Input: dimensioned drawing with shaded views. Units: mm. Origin: part minimum x, y, z. Coordinates: 2 decimals unless noted, no trailing zeros. Loops run counter-clockwise (first coordinate to the right, second up) from the corner with the lowest first, then second, coordinate; pieces in that order, holes last. Notation, with made-up numbers: (29, 4.5) - (67, 4.5) arc R22 cw to (67, 11.5) - close; hole circle Ø9 at (-2, -5). An arc over 180 degrees is marked (long way). Put each result on its own line as item: value. Start each with the question number.
1) Material intervals for line 1 along Y through (x, z) = (15.5, 6); line 2 along X through (y, z) = (7.5, 8.75); line 3 along Z through (x, y) = (13.5, 38), sorted ascending. Write a range as from..to.
2) Section B-B on z = 7.25. Output: boundary loops of the cut face in (x, y), and give its area (4 significant figures).
3) Section C-C on x = 2. Output: boundary loops of the cut face in (y, z).
4) Draft query along Z for the marked faces 1, 2 and 3. Return one class per face: +Z half, -Z half, draft (parallel to the pull), parting line (faces both ways), or undercut.
5) Section A-A on x = 9.25. Output: boundary loops of the cut face in (y, z).
6) Section D-D on z = 11. Output: boundary loops of the cut face in (x, y), and give its area (3 significant figures).
7) Contact query for flat-ended pins moving along their axis: pin 1 Ø5 at (x, z) = (18, 11.5) entering from -Y; pin 2 Ø1.5 at (x, z) = (8, 9) entering from +Y; pin 3 Ø4 at (y, z) = (6, 4) entering from -X. Output: stop coordinate, or through.
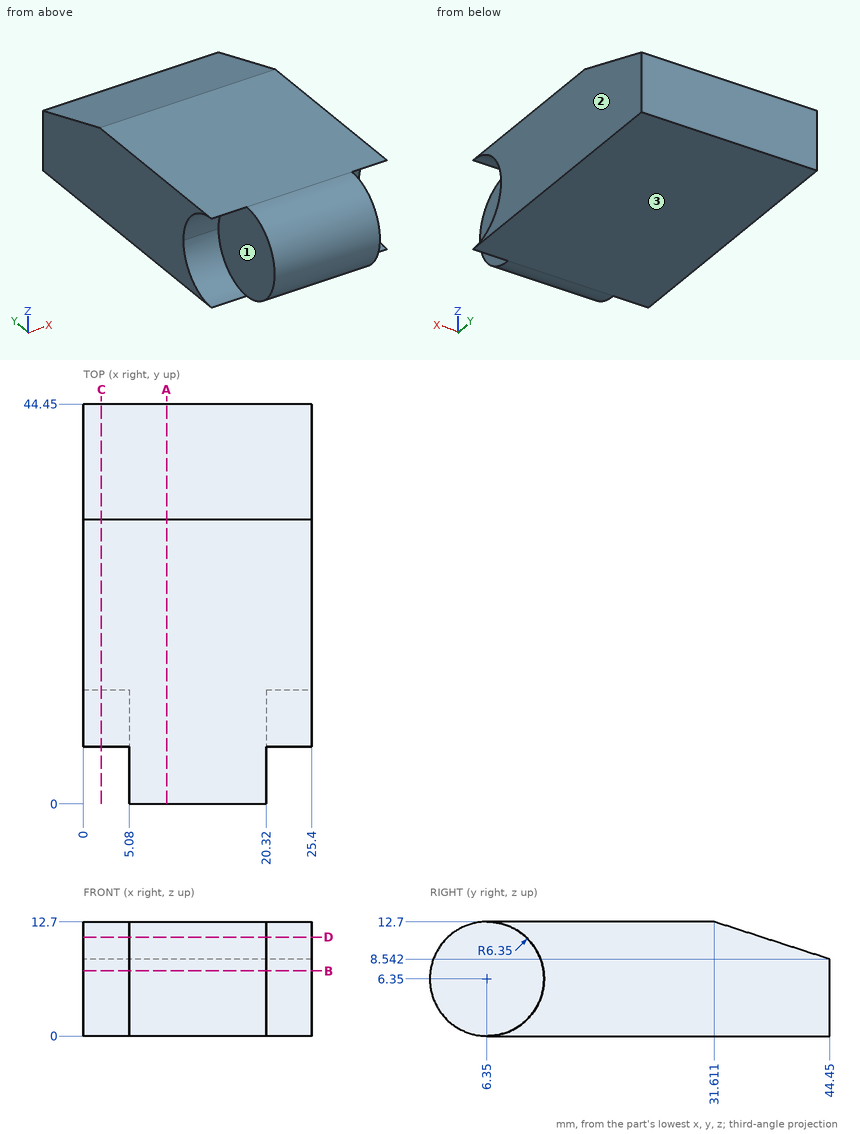
Answer block:
1. line 1: y = 0.01..44.45
1. line 2: x = 5.08..20.32
1. line 3: z = 0..10.63
2. outline: (0, 12.64) - (5.08, 12.64) - (5.08, 0.06) - (20.32, 0.06) - (20.32, 12.64) - (25.4, 12.64) - (25.4, 44.45) - (0, 44.45) - close
2. area: 1,000 mm²
3. outline: (6.35, 0) - (44.45, 0) - (44.45, 8.54) - (31.61, 12.7) - (6.35, 12.7) arc R6.35 cw to start
4. face 1: undercut
4. face 2: draft
4. face 3: -Z half
5. outline: (6.35, 0) - (44.45, 0) - (44.45, 8.54) - (31.61, 12.7) - (6.35, 12.7) arc R6.35 ccw to start
6. outline: (0, 10.67) - (5.08, 10.67) - (5.08, 2.03) - (20.32, 2.03) - (20.32, 10.67) - (25.4, 10.67) - (25.4, 36.86) - (0, 36.86) - close
6. area: 797 mm²
7. pin 1: stops at y = 0.58
7. pin 2: stops at y = 44.45
7. pin 3: stops at x = 5.08
